Design review of the part built by this model. Coordinates are the model's own, in mm. A direction names the side the tool comes from. Round coordinates to 2 decimals unless told otherwise and drop trailing zeros. Order: outer loops, then holes, each group sorted by start corner. A loop starts at its lowest first (then second) coordinate and runs counter-clockwise, first axis right, second up. Notation, with made-up numbers: (16.5, -40) - (37.5, -40) arc R32 ccw to (37.5, -11) - close; hole circle Ø5 at (-24, -1.75). An arc over 180 degrees is marked (long way). Write item = value, one per line.
from build123d import *

# Parameters (mm, degrees)
SKETCH2_R          = 3.75
CUT_EXTRUDE1_DEPTH = 500


with BuildPart() as part:
    # Sketch1 → Revolve1 (revolve)
    with BuildSketch(Plane.XY, mode=Mode.PRIVATE) as revolve1_sk:
        with BuildLine():
            Line((17.5, 0), (17.5, 7.5))
            Line((17.5, 7.5), (25, 7.5))
            ThreePointArc((25, 7.5), (17.67766953, 25.17766953), (0, 32.5))
            Line((0, 32.5), (0, 30))
            ThreePointArc((0, 30), (15, 24.270509831), (22.360679775, 10))
            Line((22.360679775, 10), (15, 10))
            Line((15, 10), (15, 0))
            Line((15, 0), (17.5, 0))
        make_face()
    revolve(revolve1_sk.sketch.rotate(Axis((0, 0, 0), (0, 1, 0)), 90), axis=Axis((0, 0, 0), (0, 1, 0)))

    # Sketch2 → Cut-Extrude1 (cut)
    with BuildSketch(Plane.XY):
        with Locations(Location((8.758891379, 20.589020037, 0), (0, 0, 229.536406865))):
            Circle(SKETCH2_R)
        with Locations(Location((-8.758891379, 20.589020037, 0), (0, 0, 238.427728908))):
            Circle(SKETCH2_R)
    extrude(amount=-CUT_EXTRUDE1_DEPTH, mode=Mode.SUBTRACT)


solid = part.part
1) We need section C-C on z = 0. Write out the cut boundary in (x, y).
Findings:
outline = (-25, 7.5) - (-17.5, 7.5) - (-17.5, 0) - (-15, 0) - (-15, 10) - (-22.36, 10) arc R22.5 cw to (22.36, 10) - (15, 10) - (15, 0) - (17.5, 0) - (17.5, 7.5) - (25, 7.5) arc R25 ccw to start
2) The part is to be moulded in two halves that separate along Y. For faces 5 (the cylindrical face through (-12.65, 4.93, -8.06)), 6 (the flat face through (5, 7.5, -17)), 7 (the cylindrical face through (-6.749, 23.755, -16.951)), say which applies: released by +Y, released by -Y, zero draft, split by the parting line, or undercut.
Findings:
face_5 = zero draft
face_6 = released by -Y
face_7 = undercut
3) We need section A-A on x = 9. Write out the cut boundary in (y, z), and give its area (3 significant figures).
Findings:
outline = (0, -15.01) - (7.5, -15.01) - (7.5, -23.32) arc R23.32 ccw to (16.85, -21.37) - (16.85, -18.38) arc R20.62 cw to (10, -20.47) - (10, -12) - (0, -12) - close; (0, 12) - (10, 12) - (10, 20.47) arc R20.62 cw to (24.33, -11.91) - (24.33, -16.15) arc R23.32 ccw to (7.5, 23.32) - (7.5, 15.01) - (0, 15.01) - close
area = 249 mm^2
4) We need section B-B on y = 20. Write out the cut boundary in (x, z).
Findings:
outline = (-12.46, -17.7) - (-12.46, -13.95) arc R18.71 cw (long way) to (12.46, -13.95) - (12.46, -17.7) arc R21.65 ccw (long way) to start; (-5.06, -21.05) arc R21.65 ccw to (5.06, -21.05) - (5.06, -18.01) arc R18.71 cw to (-5.06, -18.01) - close
5) To check wall thickness, follow L1, parallel to X at y = 6, z = 0; L2, parallel to Y at x = 3, z = -18.5; L3, parallel to Y at x = -18, z = 2. State the ranges of each line that lie inside material, in increasing order. Write a range as from..to.
Findings:
L1 = -17.5..-15, 15..17.5
L2 = 7.5..10, 19.95..24.05
L3 = 7.5..10, 20.85..24.73
6) We need section D-D on x = 0. Write out the cut boundary in (y, z), and give its area (3 significant figures).
Findings:
outline = (0, -17.5) - (7.5, -17.5) - (7.5, -25) arc R25 ccw to (7.5, 25) - (7.5, 17.5) - (0, 17.5) - (0, 15) - (10, 15) - (10, 22.36) arc R22.5 cw to (10, -22.36) - (10, -15) - (0, -15) - close
area = 261 mm^2
7) Clearance check with flat-ended pins moving along their axes: pin 1 Ø12 at (x, z) = (0.5, 16.5) entering from -Y; pin 2 Ø4.5 at (x, y) = (8.76, 20.59) entering from +Z; pin 3 Ø1.5 at (x, y) = (-8, 28) entering from +Z; pin 4 Ø8 at (y, z) = (25.5, -16.5) entering from -X. State where each tip first meets the part, or that it passes through.
Findings:
pin_1 = 0
pin_2 = 21.04
pin_3 = 13.16
pin_4 = -14.43
8) For faces 1 (the flat face through (-8, 0, 13)), 2 (the cylindrical face through (12.466, 21.156, -16.554)), 3 (the cylindrical face through (17.084, 3.802, 3.794)), 4 (the flat face through (15, 10, -5)), list the 3-axis set-ups (+Z, -Z, +X, -X, +Y, -Y) from which the entire face can be reached by the end or side of a thin tool; tool diameter is ignored.
Findings:
face_1 = +Z, -Z, +X, -X, -Y
face_2 = -Z
face_3 = -Y
face_4 = none
